Answer from the drawing. Dimensions are ordinates in mm from the lowest x, y and z of the part. A direction names the side the tool comes from. Give positions to 0.01 mm unless a question says otherwise; leave off trailing zeros. Order: outer loops, then holes, each group sorted by start corner. A loop starts at its lowest first (then second) coordinate and runs counter-clockwise, first axis right, second up.
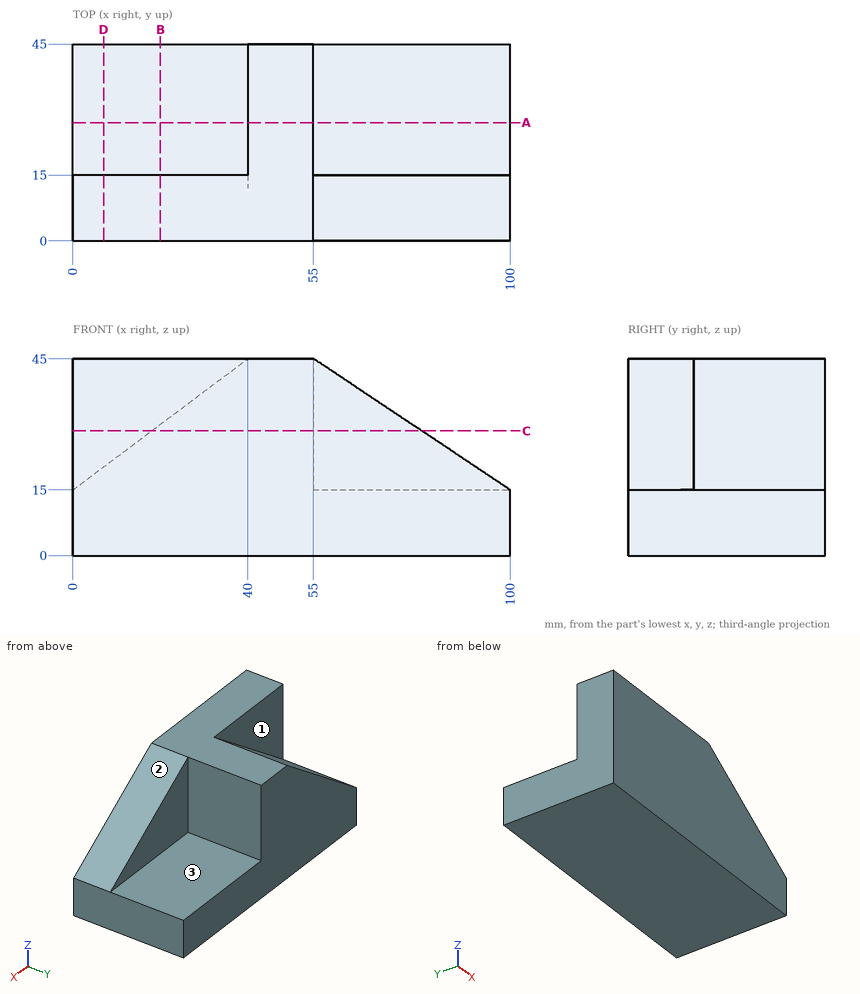
1. The part is cut by section A-A (y = 27). Write down the section's boundary in (x, z), then the cut area to 3 significant figures.
Findings below:
outline: (0, 0) - (100, 0) - (100, 15) - (55, 15) - (55, 45) - (40, 45) - (0, 15) - close
area: 2,550 mm2
2. The part is cut by section D-D (x = 7). Write down the section's boundary in (y, z), then the cut area to 3 significant figures.
Findings below:
outline: (0, 0) - (45, 0) - (45, 20.25) - (15, 20.25) - (15, 45) - (0, 45) - close
area: 1,280 mm2
3. The part is cut by section C-C (z = 28.5). Write down the section's boundary in (x, y), then the cut area to 3 significant figures.
Findings below:
outline: (0, 0) - (79.75, 0) - (79.75, 15) - (55, 15) - (55, 45) - (18, 45) - (18, 15) - (0, 15) - close
area: 2,310 mm2
4. Straight lines are drawn through the part: probe 1 along Y at (x, z) = (75, 28); probe 2 along Z at (x, y) = (22, 29). For each, find the intervals that lie inside material, in ascending order.
Findings below:
probe 1: y = 0 to 15
probe 2: z = 0 to 31.5
5. The part is cut by section B-B (x = 20). Write down the section's boundary in (y, z), then the cut area to 4 significant figures.
Findings below:
outline: (0, 0) - (45, 0) - (45, 30) - (15, 30) - (15, 45) - (0, 45) - close
area: 1,575 mm2
6. Given P1, Ø9, axis at x = 67.5, y = 29.5, coming from the +Z side; P2, Ø2, axis at x = 17.5, y = 35.5, coming from the +Z side (3 decimals); P3, Ø6, axis at y = 32.5, z = 28.5, coming from the +X side, each flat-ended and moving along its own axis, determine where each tip first touches the part or whether it passes through.
Findings below:
P1: stops at z = 15
P2: stops at z = 28.875
P3: stops at x = 55
7. Which of the six approach directions +Z, -Z, +X, -X, +Y, -Y give full straight-line access (tool end or side, diameter ignored) to the marked faces 1, 2 and 3?
Findings below:
face 1: +Z, -X, +Y
face 2: +Z, +X, +Y, -Y
face 3: +Z, +X, +Y
